Model file for the job. Use its own axes, mm. Face numbers are marked on the shaded views. A direction names the side the tool comes from. Give positions to 0.01 mm unless a question says otherwise; leave off trailing zeros. Loops run counter-clockwise (first coordinate to the right, second up) from the corner with the lowest first, then second, coordinate; pieces in that order, holes last. Notation, with made-up numbers: M -19.75,73 L 20.25,73 A15 cw 20.25,95 Z; hole C 28,-39 d8. An arc over 180 degrees is marked long. Answer in a Markdown table with one row per item.
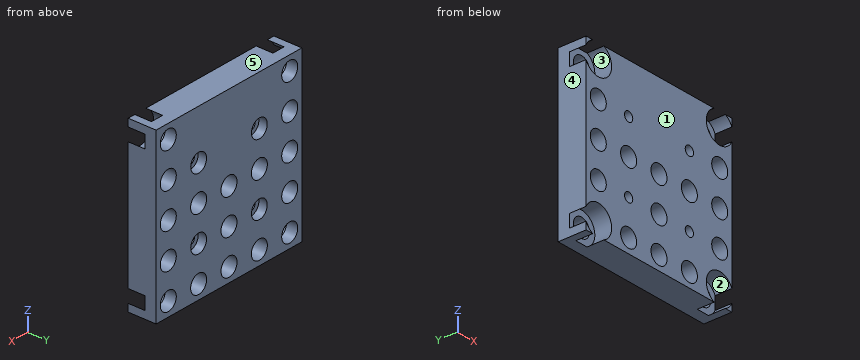
```python
from build123d import *

# Parameters (mm, degrees)
SKETCH1_W                      = 60
SKETCH1_H                      = 60
EXTRUDE1_DEPTH                 = 10
CBORE_FOR_M3_SHCS1_D           = 3.4
CBORE_FOR_M3_SHCS1_CBORE_D     = 6.5
CBORE_FOR_M3_SHCS1_CBORE_DEPTH = 3
LPATTERN2_COUNT                = 2
LPATTERN2_PITCH                = 25
LPATTERN2_COUNT_DIR2           = 2
LPATTERN2_PITCH_DIR2           = 25
CBORE_FOR_M6_SHCS1_D           = 6.6
CBORE_FOR_M6_SHCS1_CBORE_D     = 11
CBORE_FOR_M6_SHCS1_CBORE_DEPTH = 6
LPATTERN3_COUNT                = 2
LPATTERN3_PITCH                = 50
LPATTERN3_COUNT_DIR2           = 2
LPATTERN3_PITCH_DIR2           = 50
LPATTERN5_COUNT                = 2
LPATTERN5_PITCH                = 12.5
LPATTERN5_COL_COUNT            = 2
LPATTERN5_COL_PITCH            = 12.5
LPATTERN6_COUNT                = 2
LPATTERN6_PITCH                = 12.5
LPATTERN7_COUNT                = 2
LPATTERN7_PITCH                = 12.5
LPATTERN7_COL_COUNT            = 2
LPATTERN7_COL_PITCH            = 12.5
LPATTERN8_COUNT                = 3
LPATTERN8_PITCH                = 12.5
LPATTERN9_COUNT                = 2
LPATTERN9_PITCH                = 12.5
LPATTERN9_COL_COUNT            = 2
LPATTERN9_COL_PITCH            = 12.5
LPATTERN10_COUNT               = 2
LPATTERN10_PITCH               = 12.5


with BuildPart() as part:
    # Sketch1 → Extrude1 (new body)
    with BuildSketch(Plane(origin=(0, 0, 0), x_dir=(1, 0, 0), z_dir=(0, 1, 0))):
        Rectangle(SKETCH1_W, SKETCH1_H)
    extrude(amount=EXTRUDE1_DEPTH)

    # CBORE for M3 SHCS1 (through all)
    with Locations(Plane(origin=(-12.5, 10, -12.5), x_dir=(0, 0, 1), z_dir=(0, 1, 0))):
        with Locations((0, 0)):
            cbore_for_m3_shcs1 = CounterBoreHole(CBORE_FOR_M3_SHCS1_D / 2, CBORE_FOR_M3_SHCS1_CBORE_D / 2, CBORE_FOR_M3_SHCS1_CBORE_DEPTH)

    # LPattern2: CBORE for M3 SHCS1 2 × 2
    with Locations(*[(j * LPATTERN2_PITCH_DIR2, 0, i * LPATTERN2_PITCH) for i in range(LPATTERN2_COUNT) for j in range(LPATTERN2_COUNT_DIR2) if (i, j) != (0, 0)]):
        add(cbore_for_m3_shcs1, mode=Mode.SUBTRACT)

    # CBORE for M6 SHCS1 (through all)
    with Locations(Plane(origin=(25, 0, -25), x_dir=(0, 0, -1), z_dir=(0, -1, 0))):
        with Locations((0, 0)):
            cbore_for_m6_shcs1 = CounterBoreHole(CBORE_FOR_M6_SHCS1_D / 2, CBORE_FOR_M6_SHCS1_CBORE_D / 2, CBORE_FOR_M6_SHCS1_CBORE_DEPTH)

    # LPattern3: CBORE for M6 SHCS1 2 × 2
    with Locations(*[(-i * LPATTERN3_PITCH, 0, j * LPATTERN3_PITCH_DIR2) for i in range(LPATTERN3_COUNT) for j in range(LPATTERN3_COUNT_DIR2) if (i, j) != (0, 0)]):
        add(cbore_for_m6_shcs1, mode=Mode.SUBTRACT)

    # Sketch7 → M6 Clearance Hole1 (revolve, cut)
    with BuildSketch(Plane(origin=(0, 0, -25), x_dir=(0, 0, -1), z_dir=(1, 0, 0))):
        Polygon((0, 0), (0, 11.982840043), (3.3, 10), (3.3, 0), align=None)
    m6_clearance_hole1 = revolve(axis=Axis((0, -6.35, -25), (0, 1, 0)), mode=Mode.SUBTRACT)

    # LPattern5: M6 Clearance Hole1 ×2
    with Locations(*[(-i * LPATTERN5_PITCH, 0, 0) for i in range(1, LPATTERN5_COUNT)]):
        add(m6_clearance_hole1, mode=Mode.SUBTRACT)

    # LPattern5 col: M6 Clearance Hole1 ×2
    with Locations(*[(i * LPATTERN5_COL_PITCH, 0, 0) for i in range(1, LPATTERN5_COL_COUNT)]):
        add(m6_clearance_hole1, mode=Mode.SUBTRACT)

    # LPattern6: M6 Clearance Hole1 ×2
    with Locations(*[(0, 0, i * LPATTERN6_PITCH) for i in range(1, LPATTERN6_COUNT)]):
        add(m6_clearance_hole1, mode=Mode.SUBTRACT)

    # Sketch9 → M6 Clearance Hole2 (revolve, cut)
    with BuildSketch(Plane(origin=(25, 0, 0), x_dir=(0, 0, -1), z_dir=(1, 0, 0))):
        Polygon((0, 0), (0, 11.982840043), (3.3, 10), (3.3, 0), align=None)
    m6_clearance_hole2 = revolve(axis=Axis((25, -6.35, 0), (0, 1, 0)), mode=Mode.SUBTRACT)

    # LPattern7: M6 Clearance Hole2 ×2
    with Locations(*[(0, 0, i * LPATTERN7_PITCH) for i in range(1, LPATTERN7_COUNT)]):
        add(m6_clearance_hole2, mode=Mode.SUBTRACT)

    # LPattern7 col: M6 Clearance Hole2 ×2
    with Locations(*[(0, 0, -i * LPATTERN7_COL_PITCH) for i in range(1, LPATTERN7_COL_COUNT)]):
        add(m6_clearance_hole2, mode=Mode.SUBTRACT)

    # LPattern8: M6 Clearance Hole2 ×3
    with Locations(*[(-i * LPATTERN8_PITCH, 0, 0) for i in range(1, LPATTERN8_COUNT)]):
        add(m6_clearance_hole2, mode=Mode.SUBTRACT)

    # Sketch10 → M6 Clearance Hole3 (revolve, cut)
    with BuildSketch(Plane(origin=(-25, 0, 0), x_dir=(0, 0, -1), z_dir=(1, 0, 0))):
        Polygon((0, 0), (0, 11.982840043), (3.3, 10), (3.3, 0), align=None)
    m6_clearance_hole3 = revolve(axis=Axis((-25, -6.35, 0), (0, 1, 0)), mode=Mode.SUBTRACT)

    # LPattern9: M6 Clearance Hole3 ×2
    with Locations(*[(0, 0, i * LPATTERN9_PITCH) for i in range(1, LPATTERN9_COUNT)]):
        add(m6_clearance_hole3, mode=Mode.SUBTRACT)

    # LPattern9 col: M6 Clearance Hole3 ×2
    with Locations(*[(0, 0, -i * LPATTERN9_COL_PITCH) for i in range(1, LPATTERN9_COL_COUNT)]):
        add(m6_clearance_hole3, mode=Mode.SUBTRACT)

    # LPattern10: M6 Clearance Hole3 ×2
    with Locations(*[(i * LPATTERN10_PITCH, 0, 0) for i in range(1, LPATTERN10_COUNT)]):
        add(m6_clearance_hole3, mode=Mode.SUBTRACT)


solid = part.part
```
Q1. Drop flat-ended pins along their axis: pin 1 (6 mm diameter, centred on x = 25, z = -12.5, fed in from +Y); pin 2 (2 mm diameter, centred on x = -11, z = 13, fed in from +Y). Give the stop position or say it passes through.
Reported:
| item | result |
|---|---|
| pin 1 | through |
| pin 2 | y = 7 |
Q2. Saw through at B-B (y = 8.5). Give the number of separate pieces and of enclosed holes in the cut face, and give its area (3 significant figures).
Reported:
| item | result |
|---|---|
| separate pieces | 1 |
| enclosed holes | 21 |
| area | 2,890 mm² |
Q3. Probe probe 1 along X at (y, z) = (4.75, -12.5); probe 2 along X at (y, z) = (5.25, 12.5); probe 3 along X at (y, z) = (5, 0). List the from-to ranges inside material, lowest first.
Reported:
| item | result |
|---|---|
| probe 1 | -30 to -28.3, -21.7 to -14.2, -10.8 to -3.3, 3.3 to 10.8, 14.2 to 21.7, 28.3 to 30 |
| probe 2 | -30 to -28.3, -21.7 to -14.2, -10.8 to 10.8, 14.2 to 21.7, 28.3 to 30 |
| probe 3 | -30 to -28.3, -21.7 to -15.8, -9.2 to -3.3, 3.3 to 9.2, 15.8 to 21.7, 28.3 to 30 |
Q4. Saw through at D-D (z = 12.5). Give the cut face in (x, y).
Reported:
| item | result |
|---|---|
| outline | M -30,0 L -28.3,0 L -28.3,10 L -30,10 Z; M -21.7,0 L -14.2,0 L -14.2,7 L -15.75,7 L -15.75,10 L -21.7,10 Z; M -10.8,0 L 10.8,0 L 10.8,7 L 9.25,7 L 9.25,10 L -9.25,10 L -9.25,7 L -10.8,7 Z; M 14.2,0 L 21.7,0 L 21.7,10 L 15.75,10 L 15.75,7 L 14.2,7 Z; M 28.3,0 L 30,0 L 30,10 L 28.3,10 Z |
Q5. Saw through at A-A (z = -25). Give the cut face in (x, y).
Reported:
| item | result |
|---|---|
| outline | M -30,6 L -28.3,6 L -28.3,10 L -30,10 Z; M -21.7,6 L -19.5,6 L -19.5,0 L -15.8,0 L -15.8,10 L -21.7,10 Z; M -9.2,0 L -3.3,0 L -3.3,10 L -9.2,10 Z; M 3.3,0 L 9.2,0 L 9.2,10 L 3.3,10 Z; M 15.8,0 L 19.5,0 L 19.5,6 L 21.7,6 L 21.7,10 L 15.8,10 Z; M 28.3,6 L 30,6 L 30,10 L 28.3,10 Z |
Q6. Mould opens along Z. For the marked faces 3, 4 and 5 say: released by +Z, released by -Z, zero draft, split by the parting line, or undercut.
Reported:
| item | result |
|---|---|
| face 3 | undercut |
| face 4 | zero draft |
| face 5 | released by +Z |
Q7. Saw through at C-C (x = -12.5). Give the cut face in (y, z).
Reported:
| item | result |
|---|---|
| outline | M 0,-30 L 10,-30 L 10,-28.3 L 0,-28.3 Z; M 0,-21.7 L 10,-21.7 L 10,-15.75 L 7,-15.75 L 7,-14.2 L 0,-14.2 Z; M 0,-10.8 L 7,-10.8 L 7,-9.25 L 10,-9.25 L 10,-3.3 L 0,-3.3 Z; M 0,3.3 L 10,3.3 L 10,9.25 L 7,9.25 L 7,10.8 L 0,10.8 Z; M 0,14.2 L 7,14.2 L 7,15.75 L 10,15.75 L 10,30 L 0,30 Z |
Q8. 3-axis set-ups, long thin cutter, end or side, ignore diameter. For the marked faces 1 and 2: which of +Z, -Z, +X, -X, +Y, -Y reach the whole face in a straight line?
Reported:
| item | result |
|---|---|
| face 1 | +Z, -Z, +X, -X, -Y |
| face 2 | -Y |
